For this review, take the finished solid that the model builds, in its own axes (mm). A direction names the side the tool comes from. Give positions to 0.01 mm unless a question says otherwise; leave off trailing zeros. Write each loop counter-clockwise with the first axis right and the second up, starting at its lowest first coordinate (ties: lowest second). Pieces come first, ordered by that corner, then holes.
from build123d import *

# Parameters (mm, degrees)
F2_W           = 8.25
F2_H           = 22
F3_DEPTH       = 9.001
F3_DEPTH_BACK  = 9.001
F5_D           = 4.0386
F5_DEPTH       = 4.876
F6_D           = 8.35
F6_DEPTH       = 1.25
F6_TIP         = 2.5085930844
F8_D           = 8.4
F8_DEPTH       = 4.8760001
F10_DEPTH      = 9.0010001
F10_DEPTH_BACK = 9.0010001007


with BuildPart() as f1:
    # F0 (on Front) → F1 (revolve)
    with BuildSketch(Plane.XZ):
        Polygon((9, 0), (0, 0), (0, -35.7), (7.9, -35.7), (7.9, -33.7), (5.2, -33.7), (5.2, -27.85), (7.9, -27.85), (7.9, -22.7), (9, -22.7), align=None)
    revolve(axis=Axis((0, 0, -17.85), (0, 0, 1)))

    # F2 (on Right) → F3 (cut, two sides)
    with BuildSketch(Plane.YZ) as f3_sk:
        with Locations((0, -11)):
            Rectangle(F2_W, F2_H)
    extrude(amount=-F3_DEPTH, mode=Mode.SUBTRACT)
    extrude(f3_sk.sketch, amount=F3_DEPTH_BACK, mode=Mode.SUBTRACT)

    # F5 (through all, one way)
    with BuildSketch(Plane(origin=(0, -4.125, 0), x_dir=(-1, 0, 0), z_dir=(0, 1, 0))):
        with Locations((0, -8)):
            Circle(F5_D / 2)
    extrude(amount=-F5_DEPTH, mode=Mode.SUBTRACT)

    # F6 (one way)
    with BuildSketch(Plane(origin=(0, -4.125, 0), x_dir=(-1, 0, 0), z_dir=(0, 1, 0))):
        with Locations((0, -8)):
            Circle(F6_D / 2)
    extrude(amount=-F6_DEPTH, mode=Mode.SUBTRACT)
    with Locations(Plane(origin=(0, -4.125, 0), x_dir=(-1, 0, 0), z_dir=(0, 1, 0))):
        with Locations((0, -8)):
            with Locations((0, 0, -(F6_DEPTH + F6_TIP / 2))):  # 118° drill point
                Cone(0, F6_D / 2, F6_TIP, mode=Mode.SUBTRACT)

    # F8 (through all, one way)
    with BuildSketch(Plane.XZ.offset(-4.125)):
        with Locations((0, -8)):
            Circle(F8_D / 2)
    extrude(amount=-F8_DEPTH, mode=Mode.SUBTRACT)

    # F9 (on Front) → F10 (cut, two sides)
    with BuildSketch(Plane.XZ) as f10_sk:
        with BuildLine():
            ThreePointArc((-8, -8), (0, 0), (8, -8))
            Line((8, -8), (8, 2.4616862277))
            Line((8, 2.4616862277), (-8, 2.4616862277))
            Line((-8, 2.4616862277), (-8, -8))
        make_face()
    extrude(amount=-F10_DEPTH, mode=Mode.SUBTRACT)
    extrude(f10_sk.sketch, amount=F10_DEPTH_BACK, mode=Mode.SUBTRACT)


solid = f1.part
(1) Tool access review of faces 1 (the flat face through (2, -5, -33.7)), 2 (the cylindrical face through (-6.269, -4.807, -34.686)), 3 (the cylindrical face through (-4.196, 6.528, -7.815)), 4 (the cylindrical face through (0, -6, 0)), 5 (the flat face through (0, 0, -22)): name each direction out of +Z, -Z, +X, -X, +Y, -Y from which nothing blocks a thin tool from reaching the whole face with its end or side.
(2) For L1, parallel to Z at x = -3.75, y = 6; L2, parallel to Z at x = 1.25, y = -2.25; L3, parallel to Z at x = 0, y = -4.95 (3 decimals), list the stretches that pass through material, from the lowest coordinate up.
(3) The part is to be moulded in two halves that separate along X. For faces 6 (the cylindrical face through (0.263, -7.822, -5.998)), 7 (the cylindrical face through (0, 6, 0)), 8 (the flat face through (0, 0, -35.7)), say which applies: +X half, -X half, draft (parallel to the pull), parting line (faces both ways), or undercut.
(4) We need section D-D (z = -18). Write out the cut boundary in (x, y) (3 decimals).
(5) We need section A-A (x = 0). Count the separate pieces of the cut face and the enclosed holes in it, and give its area (3 significant figures).
(6) We need section B-B (y = 7.5). Write out the cut boundary in (x, z), and give its area (3 significant figures).
(7) Clearance check with flat-ended pins moving along their axes: pin 1 Ø5.5 at (x, z) = (0, -8) entering from +Y; pin 2 Ø10 at (x, z) = (5.5, -22) entering from -Y; pin 3 Ø2.5 at (x, y) = (-3.5, 0.5) entering from +Z; pin 4 Ø8 at (x, y) = (3.5, 3) entering from +Z. State where each tip first meets the part, or that it passes through.
The answers:
1. face 1: none
1. face 2: -Z
1. face 3: +Y
1. face 4: +Z, +Y, -Y
1. face 5: +Z, +X, -X
2. L1: z = -35.7 to -33.7, -27.85 to -9.89, -6.11 to -0.93
2. L2: z = -35.7 to -22
2. L3: z = -35.7 to -12.175, -3.825 to 0
3. face 6: undercut
3. face 7: parting line
3. face 8: draft
4. outline: (-7.999, -4.125) arc R9 ccw to (7.999, -4.125) - close; (-7.999, 4.125) - (7.999, 4.125) arc R9 ccw to start
5. separate pieces: 3
5. enclosed holes: 0
5. area: 332 mm2
6. outline: (-4.97, -22.7) - (-2.48, -22.7) - (-2.48, -27.85) - (2.48, -27.85) - (2.48, -22.7) - (4.97, -22.7) - (4.97, -1.74) arc R8 ccw to (-4.97, -1.74) - close; (-2.48, -35.7) - (2.48, -35.7) - (2.48, -33.7) - (-2.48, -33.7) - close; hole circle Ø8.4 at (0, -8)
6. area: 200 mm2
7. pin 1: stops at y = -6.23
7. pin 2: stops at y = -8.99
7. pin 3: stops at z = -22
7. pin 4: stops at z = 0
